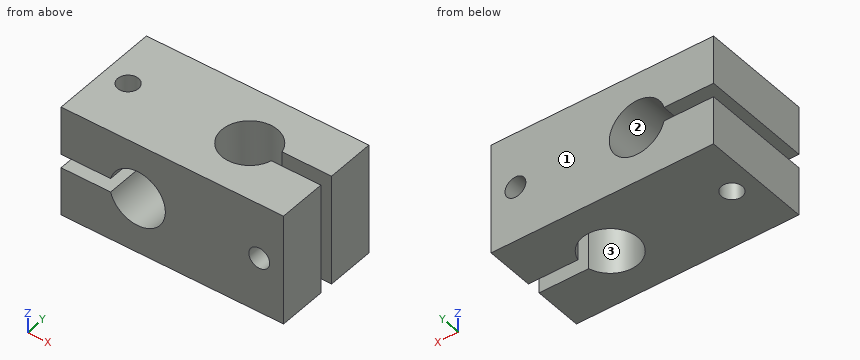
Autodesk Inventor part; units mm, degrees
ref_plane "YZ Plane" through (0, 0, 0) normal (1, 0, 0) x (0, 1, 0)
ref_plane "XZ Plane" through (0, 0, 0) normal (0, 1, 0) x (-1, 0, 0)
ref_plane "XY Plane" through (0, 0, 0) normal (0, 0, 1) x (1, 0, 0)
sketch "Sketch1" plane through (0, 0, 0) normal (1, 0, 0) x (0, 1, 0)
  line L0 (0, 0) -> (16, 0)
  line L1 (16, 0) -> (16, 16)
  line L2 (16, 16) -> (0, 16)
  line L3 (0, 16) -> (0, 0)
  dimension "d0" = 16
  dimension "d1" = 16
extrude "Extrusion1" add sketch "Sketch1" along normal blind 32
sketch "Sketch2" plane through (0, 0, 16) normal (0, 0, 1) x (1, 0, 0)
  line L0 (32, 16) -> (32, 0)
  circle A0 centre (21, 8) radius 4
  line L1 (32, 8) -> (32, 9)
  line L2 (32, 9) -> (32, 7)
  line L3 (32, 7) -> (24.873, 7)
  line L4 (32, 9) -> (24.873, 9)
  circle A1 centre (3.5, 8) radius 1.5
  dimension "d5" = 8
  dimension "d6" = 1
  dimension "d7" = 2
  dimension "d9" = 3
extrude "Extrusion2" cut sketch "Sketch2" against normal blind 32
sketch "Sketch3" plane through (0, 16, 16) normal (0, 1, 0) x (1, 0, 0)
  line L0 (0, 16) -> (0, 0)
  line L1 (0, 0) -> (32, 0)
  line L2 (32, 16) -> (32, 0)
  line L3 (0, 16) -> (32, 16)
  line L4 (16, 16) -> (16, 0)
  line L5 (16, 8) -> (11, 8)
  circle A0 centre (11, 8) radius 4
  line L6 (0, 8) -> (0, 9)
  line L7 (0, 9) -> (7.127, 9)
  line L8 (0, 8) -> (0, 7)
  line L9 (0, 7) -> (7.127, 7)
  line L10 (32, 8) -> (28.5, 8)
  circle A1 centre (28.5, 8) radius 1.5
  dimension "d12" = 5
  dimension "d13" = 8
  dimension "d14" = 1
  dimension "d15" = 1
  dimension "d16" = 3.5
  dimension "d17" = 3
extrude "Extrusion3" cut sketch "Sketch3" against normal blind 32 contours L7 A0 L9 L0 | A1 | A0
properties part number "BarClamp_V2" material "Birch"
Model file for the job. Use its own axes, mm. Face numbers are marked on the shaded views. Coordinates: 2 decimals unless noted, no trailing zeros. Order: outer loops, then holes, each group sorted by start corner. A loop starts at its lowest first (then second) coordinate and runs counter-clockwise, first axis right, second up. Notation, with made-up numbers: (44.25, 8.5) - (84.25, 8.5) arc R16 cw to (84.25, 27.5) - close; hole circle Ø10 at (-39.75, 88.25). An arc over 180 degrees is marked (long way). Return JSON: item names as keys, results as strings. Group by question number.
1) Saw through at A-A, the plane x = 30.5. Write the cut outline in (y, z), plus the area to 3 significant figures.
2) Saw through at D-D, the plane y = 8. Write the cut outline in (x, z).
3) Saw through at C-C, the plane z = 11. Write the cut outline in (x, y), plus the area to 3 significant figures.
4) Probe line 1 (Z direction, x = 28.5, y = 0.5); line 2 (Y direction, x = 25, z = 2.5); line 3 (X direction, y = 10.75, z = 8). List the from-to ranges inside material, lowest first. Write a range as from..to.
5) Saw through at B-B, the plane y = 5.75. Write the cut outline in (x, z).
6) Mould opens along Y. For the marked faces 1, 2 and 3 say: released by +Y, released by -Y, zero draft, split by the parting line, or undercut.
Values found:
{
 "1": {"outline": "(0, 0) - (7, 0) - (7, 16) - (0, 16) - close; (9, 0) - (16, 0) - (16, 16) - (9, 16) - close", "area": "224 mm²"},
 "2": {"outline": "(0, 0) - (2, 0) - (2, 7) - (0, 7) - close; (0, 9) - (2, 9) - (2, 16) - (0, 16) - close; (5, 0) - (17, 0) - (17, 16) - (5, 16) - (5, 9) - (7.13, 9) arc R4 cw (long way) to (7.13, 7) - (5, 7) - close"},
 "3": {"outline": "(0, 0) - (8.35, 0) - (8.35, 16) - (0, 16) - close; (13.65, 0) - (32, 0) - (32, 7) - (24.87, 7) arc R4 cw (long way) to (24.87, 9) - (32, 9) - (32, 16) - (13.65, 16) - close; hole circle Ø3 at (3.5, 8)", "area": "356 mm²"},
 "4": {"line 1": "z = 0..6.5, 9.5..16", "line 2": "y = 0..7, 9..16", "line 3": "x = 15..18.1, 23.9..27, 30..32"},
 "5": {"outline": "(0, 0) - (17.69, 0) - (17.69, 16) - (0, 16) - (0, 9) - (7.13, 9) arc R4 cw (long way) to (7.13, 7) - (0, 7) - close; (24.31, 0) - (32, 0) - (32, 16) - (24.31, 16) - close; hole circle Ø3 at (28.5, 8)"},
 "6": {"face 1": "released by +Y", "face 2": "zero draft", "face 3": "undercut"}
}
